from build123d import *

# Parameters (mm, degrees)
SKETCH1_R               = 60
BOSS_EXTRUDE1_DEPTH     = 7
CUT_EXTRUDE1_DEPTH      = 86.141059425
CUT_EXTRUDE1_DEPTH_BACK = 20
SKETCH7_R               = 13.442894491
CUT_EXTRUDE2_DEPTH      = 20
CUT_EXTRUDE3_DEPTH      = 4
CUT_EXTRUDE3_DEPTH_BACK = 2
SKETCH9_R               = 3.5
SKETCH13_R              = 2
CUT_EXTRUDE4_DEPTH      = 86.141059425
SKETCH14_R              = 3
CUT_EXTRUDE5_DEPTH      = 3
SKETCH15_R              = 2.45
CUT_EXTRUDE6_DEPTH      = 85.947042326
SKETCH16_R              = 3
CUT_EXTRUDE7_DEPTH      = 3
SKETCH17_R              = 2.45
CUT_EXTRUDE8_DEPTH      = 86.141059425
CUT_EXTRUDE9_DEPTH      = 1
FILLET2_R               = 0.005


with BuildPart() as part:
    # Sketch1 → Boss-Extrude1 (new body)
    with BuildSketch(Plane(origin=(0, 0, 0), x_dir=(1, 0, 0), z_dir=(0, 1, 0))):
        with Locations(Location((0, 0, 0), (0, 0, 270))):
            Circle(SKETCH1_R)
    extrude(amount=BOSS_EXTRUDE1_DEPTH)

    # Sketch5 → Cut-Extrude1 (cut, two sides: drawn at the far end of the back side and taken through both)
    with BuildSketch(Plane(origin=(0, 0, 0), x_dir=(1, 0, 0), z_dir=(0, 1, 0)).offset(-CUT_EXTRUDE1_DEPTH_BACK)):
        Polygon((-12.468903546, 50.167122687), (-28.724188041, 42.022350038), (-29.575349406, 38.302005643), (-18.186693565, 23.520652463), (-13.673554926, 22.488111162), (-5.8318542, 26.41722539), (-3.957136141, 30.650426793), (-8.979321601, 48.621724378), align=None)
        Polygon((-22.488111162, 13.673554926), (-26.41722539, 5.8318542), (-30.650426793, 3.957136141), (-48.621724378, 8.979321601), (-50.167122687, 12.468903546), (-42.022350038, 28.724188041), (-38.302005643, 29.575349406), (-23.520652463, 18.186693565), align=None)
        Polygon((22.488111162, 13.673554926), (26.41722539, 5.8318542), (30.650426793, 3.957136141), (48.621724378, 8.979321601), (50.167122687, 12.468903546), (42.022350038, 28.724188041), (38.302005643, 29.575349406), (23.520652463, 18.186693565), align=None)
        Polygon((13.673554926, 22.488111162), (5.8318542, 26.41722539), (3.957136141, 30.650426793), (8.979321601, 48.621724378), (12.468903546, 50.167122687), (28.724188041, 42.022350038), (29.575349406, 38.302005643), (18.186693565, 23.520652463), align=None)
        Polygon((22.488111162, -13.673554926), (26.41722539, -5.8318542), (30.650426793, -3.957136141), (48.621724378, -8.979321601), (50.167122687, -12.468903546), (42.022350038, -28.724188041), (38.302005643, -29.575349406), (23.520652463, -18.186693565), align=None)
        Polygon((13.673554926, -22.488111162), (5.8318542, -26.41722539), (3.957136141, -30.650426793), (8.979321601, -48.621724378), (12.468903546, -50.167122687), (28.724188041, -42.022350038), (29.575349406, -38.302005643), (18.186693565, -23.520652463), align=None)
        Polygon((-13.673554926, -22.488111162), (-5.8318542, -26.41722539), (-3.957136141, -30.650426793), (-8.979321601, -48.621724378), (-12.468903546, -50.167122687), (-28.724188041, -42.022350038), (-29.575349406, -38.302005643), (-18.186693565, -23.520652463), align=None)
        Polygon((-22.488111162, -13.673554926), (-26.41722539, -5.8318542), (-30.650426793, -3.957136141), (-48.621724378, -8.979321601), (-50.167122687, -12.468903546), (-42.022350038, -28.724188041), (-38.302005643, -29.575349406), (-23.520652463, -18.186693565), align=None)
    extrude(amount=CUT_EXTRUDE1_DEPTH + CUT_EXTRUDE1_DEPTH_BACK, mode=Mode.SUBTRACT)

    # Sketch7 → Cut-Extrude2 (cut)
    with BuildSketch(Plane(origin=(0, 7, 0), x_dir=(1, 0, 0), z_dir=(0, 1, 0))):
        with Locations(Location((0, 0, 0), (0, 0, 270))):
            Circle(SKETCH7_R)
    extrude(amount=-CUT_EXTRUDE2_DEPTH, mode=Mode.SUBTRACT)

    # Sketch9 → Cut-Extrude3 (cut, two sides: drawn at the far end of the back side and taken through both)
    with BuildSketch(Plane(origin=(0, 0, 0), x_dir=(1, 0, 0), z_dir=(0, 1, 0)).offset(-CUT_EXTRUDE3_DEPTH_BACK)):
        with Locations(Location((0, 17.8, 0), (0, 0, 270))):
            Circle(SKETCH9_R)
        with Locations(Location((17.8, 0, 0), (0, 0, 270))):
            Circle(SKETCH9_R)
        with Locations(Location((0, -17.8, 0), (0, 0, 90))):
            Circle(SKETCH9_R)
        with Locations(Location((-17.8, 0, 0), (0, 0, 90))):
            Circle(SKETCH9_R)
    extrude(amount=CUT_EXTRUDE3_DEPTH + CUT_EXTRUDE3_DEPTH_BACK, mode=Mode.SUBTRACT)

    # Sketch13 → Cut-Extrude4 (cut, through all)
    with BuildSketch(Plane(origin=(0, 0, 0), x_dir=(-1, 0, 0), z_dir=(0, -1, 0))):
        with Locations(Location((0, -17.8, 0), (0, 0, 90))):
            Circle(SKETCH13_R)
        with Locations(Location((-17.8, 0, 0), (0, 0, 90))):
            Circle(SKETCH13_R)
        with Locations(Location((0, 17.8, 0), (0, 0, 270))):
            Circle(SKETCH13_R)
        with Locations(Location((17.8, 0, 0), (0, 0, 90))):
            Circle(SKETCH13_R)
    extrude(amount=-CUT_EXTRUDE4_DEPTH, mode=Mode.SUBTRACT)

    # Sketch14 → Cut-Extrude5 (cut)
    with BuildSketch(Plane(origin=(0, 0, 0), x_dir=(-1, 0, 0), z_dir=(0, -1, 0))):
        with Locations(Location((12.374368671, -12.374368671, 0), (0, 0, 270))):
            Circle(SKETCH14_R)
        with Locations(Location((-12.374368671, -12.374368671, 0), (0, 0, 270))):
            Circle(SKETCH14_R)
        with Locations(Location((-12.374368671, 12.374368671, 0), (0, 0, 270))):
            Circle(SKETCH14_R)
        with Locations(Location((12.374368671, 12.374368671, 0), (0, 0, 270))):
            Circle(SKETCH14_R)
    extrude(amount=-CUT_EXTRUDE5_DEPTH, mode=Mode.SUBTRACT)

    # Sketch15 → Cut-Extrude6 (cut, through all)
    with BuildSketch(Plane(origin=(0, 3, 0), x_dir=(-1, 0, 0), z_dir=(0, -1, 0))):
        with Locations(Location((-12.374368671, -12.374368671, 0), (0, 0, 90))):
            Circle(SKETCH15_R)
        with Locations(Location((12.374368671, -12.374368671, 0), (0, 0, 90))):
            Circle(SKETCH15_R)
        with Locations(Location((12.374368671, 12.374368671, 0), (0, 0, 90))):
            Circle(SKETCH15_R)
        with Locations(Location((-12.374368671, 12.374368671, 0), (0, 0, 90))):
            Circle(SKETCH15_R)
    extrude(amount=-CUT_EXTRUDE6_DEPTH, mode=Mode.SUBTRACT)

    # Sketch16 → Cut-Extrude7 (cut)
    with BuildSketch(Plane(origin=(0, 0, 0), x_dir=(-1, 0, 0), z_dir=(0, -1, 0))):
        with Locations(Location((-51.552477914, 21.353735526, 0), (0, 0, 270))):
            Circle(SKETCH16_R)
        with Locations(Location((-51.552477914, -21.353735526, 0), (0, 0, 270))):
            Circle(SKETCH16_R)
        with Locations(Location((51.552477914, 21.353735526, 0), (0, 0, 270))):
            Circle(SKETCH16_R)
        with Locations(Location((51.552477914, -21.353735526, 0), (0, 0, 270))):
            Circle(SKETCH16_R)
        with Locations(Location((0, 55.8, 0), (0, 0, 270))):
            Circle(SKETCH16_R)
        with Locations(Location((0, -55.8, 0), (0, 0, 270))):
            Circle(SKETCH16_R)
    extrude(amount=-CUT_EXTRUDE7_DEPTH, mode=Mode.SUBTRACT)

    # Sketch17 → Cut-Extrude8 (cut, through all)
    with BuildSketch(Plane.XZ):
        with Locations(Location((-51.552477914, 21.353735526, 0), (0, 0, 270))):
            Circle(SKETCH17_R)
        with Locations(Location((-51.552477914, -21.353735526, 0), (0, 0, 90))):
            Circle(SKETCH17_R)
        with Locations(Location((51.552477914, -21.353735526, 0), (0, 0, 270))):
            Circle(SKETCH17_R)
        with Locations(Location((51.552477914, 21.353735526, 0), (0, 0, 90))):
            Circle(SKETCH17_R)
        with Locations(Location((0, -55.8, 0), (0, 0, 270))):
            Circle(SKETCH17_R)
        with Locations(Location((0, 55.8, 0), (0, 0, 90))):
            Circle(SKETCH17_R)
    extrude(amount=-CUT_EXTRUDE8_DEPTH, mode=Mode.SUBTRACT)

    # Sketch18 → Cut-Extrude9 (cut)
    with BuildSketch(Plane.XZ):
        with BuildLine():
            Line((3.004044194, 48.113779502), (3.004044194, 35.332130299))
            ThreePointArc((3.004044194, 35.332130299), (0, 32.328086105), (-3.004044194, 35.332130299))
            Line((-3.004044194, 35.332130299), (-3.004044194, 48.113779502))
            ThreePointArc((-3.004044194, 48.113779502), (0, 51.117823696), (3.004044194, 48.113779502))
        make_face()
        with BuildLine():
            Line((3.004044194, -48.113779502), (3.004044194, -35.332130299))
            ThreePointArc((3.004044194, -35.332130299), (0, -32.328086105), (-3.004044194, -35.332130299))
            Line((-3.004044194, -35.332130299), (-3.004044194, -48.113779502))
            ThreePointArc((-3.004044194, -48.113779502), (0, -51.117823696), (3.004044194, -48.113779502))
        make_face()
    extrude(amount=-CUT_EXTRUDE9_DEPTH, mode=Mode.SUBTRACT)

    # Fillet2
    fillet2_edges = [part.edges().sort_by_distance(p)[0] for p in [
        (0, 0, 32.328086105),
        (-3.004044194, 1, 41.7229549),
        (0, 0, 51.117823696),
        (3.004044194, 1, 41.7229549),
        (0, 1, 32.328086105),
        (0, 1, 51.117823696),
        (3.004044194, 0, 41.7229549),
        (-3.004044194, 0, 41.7229549),
    ]]
    fillet(fillet2_edges, radius=FILLET2_R)


solid = part.part
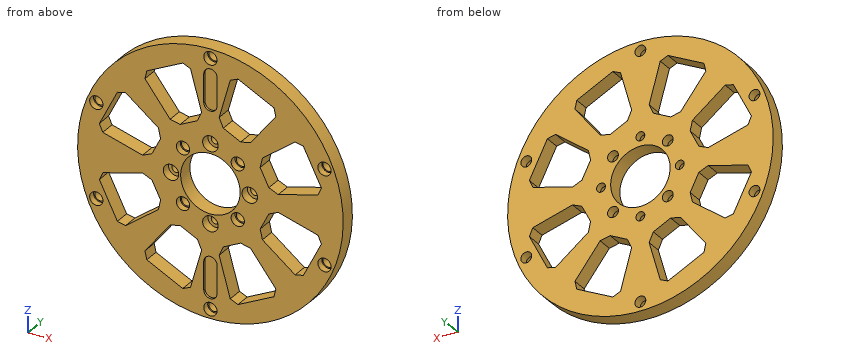
The listing builds one solid part. Answer for the finished solid, in the listing's coordinates (mm). Round coordinates to 2 decimals unless told otherwise and drop trailing zeros. Order: outer loops, then holes, each group sorted by start corner. A loop starts at its lowest first (then second) coordinate and runs counter-clockwise, first axis right, second up. Notation, with made-up numbers: M -34.5,-12 L 22.5,-12 A23 cw 22.5,27 Z; hole C 85.25,-1.5 d10. An arc over 180 degrees is marked long. Answer in a Markdown table with one row per item. Add a question column.
1) Flat-ended cylindrical pins translate along their axes: pin 1 Ø1.5 at (y, z) = (4, 47.5) entering from +X; pin 2 Ø5.5 at (x, z) = (51.55, -21.35) entering from -Y; pin 3 Ø4.5 at (x, z) = (0, -55.8) entering from +Y; pin 4 Ø7.5 at (x, z) = (-1.5, 18.5) entering from -Y. Find the tip coordinate at first contact, or state that the pin passes through.
2) The part is cut by section B-B on z = 55.8. Determine the outline of the cut face in (x, y).
3) The part is cut by section A-A on z = 0. Determine the outline of the cut face in (x, y).
4) Consider line 1 along X through (y, z) = (3, 0); line 2 along X through (y, z) = (2.05, 17.8); line 3 along Z through (x, y) = (-15.5, 6.75). Determine where each line is inside the solid, lowest interval first. Write a range as from..to.
Findings below:
| question | item | result |
|---|---|---|
| 1 | pin 1 | stops at x = 37.61 |
| 1 | pin 2 | stops at y = 3 |
| 1 | pin 3 | passes through |
| 1 | pin 4 | stops at y = 0 |
| 2 | outline | M -22.05,0 L -3,0 L -3,3 L -2.45,3 L -2.45,7 L -22.05,7 Z; M 2.45,3 L 3,3 L 3,0 L 22.05,0 L 22.05,7 L 2.45,7 Z |
| 3 | outline | M -60,0 L -21.3,0 L -21.3,4 L -19.8,4 L -19.8,7 L -60,7 Z; M -15.8,4 L -14.3,4 L -14.3,0 L -13.44,0 L -13.44,7 L -15.8,7 Z; M 13.44,0 L 14.3,0 L 14.3,4 L 15.8,4 L 15.8,7 L 13.44,7 Z; M 19.8,4 L 21.3,4 L 21.3,0 L 60,0 L 60,7 L 19.8,7 Z |
| 4 | line 1 | x = -60..-21.3, -14.3..-13.44, 13.44..14.3, 21.3..60 |
| 4 | line 2 | x = -57.3..-47.5, -23.43..-3.5, 3.5..23.43, 47.5..57.3 |
| 4 | line 3 | z = -57.96..-48.65, -22.91..22.91, 48.65..57.96 |
